from build123d import *

# Parameters (mm, degrees)
CUT_EXTRUDE1_DEPTH       = 138.249772313
CUT_EXTRUDE1_DEPTH_BACK  = 138.249772313
SKETCH3_W                = 40.4
SKETCH3_H                = 18
CUT_EXTRUDE2_REACH       = 138.463
BOSS_EXTRUDE1_DEPTH      = 2
BOSS_EXTRUDE1_DEPTH_BACK = 2
SKETCH5_R                = 8
BOSS_EXTRUDE2_DEPTH      = 2
BOSS_EXTRUDE2_DEPTH_BACK = 2
SKETCH6_R                = 8


with BuildPart() as part:
    # Sketch1 → Revolve2 (revolve)
    with BuildSketch(Plane.XY, mode=Mode.PRIVATE) as revolve2_sk:
        Polygon((-135, 5), (-26.2, 5), (-26.2, 17.5), (26.2, 17.5), (26.2, 5), (108, 5), (108, 0), (20.2, 0), (20.2, 15), (-20.2, 15), (-20.2, 0), (-135, 0), align=None)
    revolve(revolve2_sk.sketch.rotate(Axis((-109.707215801, 0, 0), (1, 0, 0)), 90), axis=Axis((-109.707215801, 0, 0), (1, 0, 0)))

    # Sketch3 → Cut-Extrude1 (cut, two sides: drawn at the far end of the back side and taken through both)
    with BuildSketch(Plane.XY.offset(-CUT_EXTRUDE1_DEPTH_BACK)):
        with Locations((0, 9)):
            Rectangle(SKETCH3_W, SKETCH3_H)
    extrude(amount=CUT_EXTRUDE1_DEPTH + CUT_EXTRUDE1_DEPTH_BACK, mode=Mode.SUBTRACT)

    # Cut-Extrude2: up to this face of the body (flat: up to its plane)
    cut_extrude2_end = Plane(part.part.faces().sort_by_distance((26.2, 0, -17.005025253))[0])
    # Sketch4 → Cut-Extrude2 (cut, up to the picked face)
    with BuildSketch(Plane.ZY.offset(26.2), mode=Mode.PRIVATE) as cut_extrude2_sk1:
        with BuildLine():
            Line((-10, 14.361406616), (-10, 11.861406616))
            Line((-10, 11.861406616), (10, 11.861406616))
            Line((10, 11.861406616), (10, 14.361406616))
            ThreePointArc((10, 14.361406616), (0, 17.5), (-10, 14.361406616))
        make_face()
    cut_extrude2_tool1 = split(extrude(cut_extrude2_sk1.sketch, amount=-CUT_EXTRUDE2_REACH, mode=Mode.PRIVATE), bisect_by=cut_extrude2_end, keep=Keep.BOTH, mode=Mode.PRIVATE)
    add(cut_extrude2_tool1.solids().sort_by(Axis((-26.2, 14.269595, 0), (1, 0, 0)))[0], mode=Mode.SUBTRACT)

    # Sketch5 → Boss-Extrude1 (add, two sides: drawn at the far end of the back side and taken through both)
    with BuildSketch(Plane(origin=(60, 0, 0), x_dir=(0, 0, -1), z_dir=(1, 0, 0)).offset(-BOSS_EXTRUDE1_DEPTH_BACK)):
        Circle(SKETCH5_R)
    extrude(amount=BOSS_EXTRUDE1_DEPTH + BOSS_EXTRUDE1_DEPTH_BACK)

    # Sketch6 → Boss-Extrude2 (add, two sides: drawn at the far end of the back side and taken through both)
    with BuildSketch(Plane(origin=(-60, 0, 0), x_dir=(0, 0, -1), z_dir=(1, 0, 0)).offset(-BOSS_EXTRUDE2_DEPTH_BACK)):
        Circle(SKETCH6_R)
    extrude(amount=BOSS_EXTRUDE2_DEPTH + BOSS_EXTRUDE2_DEPTH_BACK)


solid = part.part
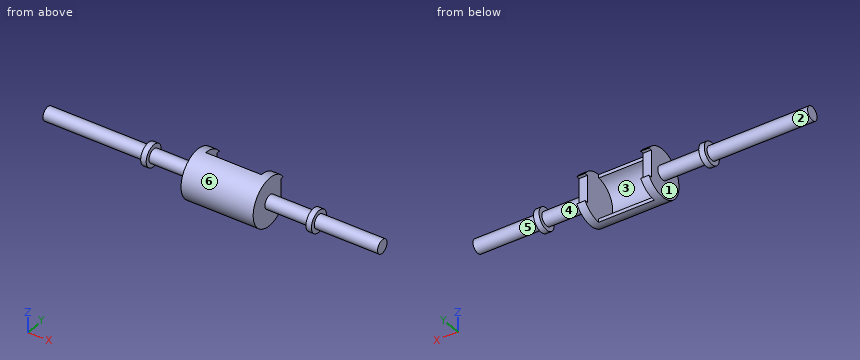
Verification items for the finished model (mm, model axes). Face numbers are marked on the shaded views. A direction names the side the tool comes from. Coordinates: 2 decimals unless noted, no trailing zeros. Loops run counter-clockwise (first coordinate to the right, second up) from the corner with the lowest first, then second, coordinate; pieces in that order, holes last. Notation, with made-up numbers: M 63.5,15.25 L 86.5,15.25 A33 ccw 86.5,43.25 Z; hole C 48.5,62 d5. An arc over 180 degrees is marked long. One line per item, written item: value.
1. Material ranges on line 1 along X through (y, z) = (2, -6.5); line 2 along X through (y, z) = (1, 14); line 3 along X through (y, z) = (0.5, 4), recorded low to high. Write a range as from..to.
Answers follow:
line 1: -62..-58, -26.2..-20.2, 20.2..26.2, 58..62
line 2: -26.2..-20.2, 20.2..26.2
line 3: -135..-20.2, 20.2..108
2. Section check D-D on x = 60. Record the cut outline in (y, z), plus the area to 3 significant figures.
Answers follow:
outline: C 0,0 d16
area: 201 mm^2
3. Gauge pin test, flat ends, axial feed: P1, Ø6.5, axis at x = -24.5, z = 3.5, coming from the +Y side; P2, Ø2, axis at x = 53, y = -5.5, coming from the -Z side; P3, Ø6, axis at x = -58.5, y = 8.5, coming from the +Z side. Record the tip position at first contact, or that the pin passes through.
Answers follow:
P1: y = 11.86
P2: z = -2.18
P3: z = 5.81
4. Set-up check for the marked faces 3, 4, 5 and 6: record each of +Z, -Z, +X, -X, +Y, -Y from which the full face is reachable in a straight line by a thin tool's end or side.
Answers follow:
face 3: +Y
face 4: none
face 5: +X
face 6: +X, -X
5. Section check C-C on z = -12. Record the cut outline in (x, y).
Answers follow:
outline: M -26.2,-12.74 L 26.2,-12.74 L 26.2,12.74 L 20.2,12.74 L 20.2,-9 L -20.2,-9 L -20.2,12.74 L -26.2,12.74 Z
6. Section check B-B on x = -74.5. Record the cut outline in (y, z), plus the area to 3 significant figures.
Answers follow:
outline: C 0,0 d10
area: 78.5 mm^2
7. Mould release check, pull along X, two halves, no side actions. Record for the marked faces 1 and 2: pulls with the +X half, pulls with the -X half, needs draft (parallel to the pull), parting line crosses it, or undercut.
Answers follow:
face 1: undercut
face 2: needs draft
